For this review, take the finished solid that the model builds, in its own axes (mm). Coordinates: 2 decimals unless noted, no trailing zeros. Order: outer loops, then holes, each group sorted by start corner. A loop starts at its lowest first (then second) coordinate and runs counter-clockwise, first axis right, second up. Notation, with made-up numbers: M -17,-21 L 41,-21 A13 cw 41,-10 Z; hole C 68.25,-34 d5. An arc over 180 degrees is marked long. Use one line per item in the form item = value. Start each with the question number.
```python
from build123d import *

# Parameters (mm, degrees)
ESBO_O1_R                = 16
RESSALTO_EXTRUS_O1_DEPTH = 6
ESBO_O2_R                = 3
ESBO_O2_W                = 55
ESBO_O2_H                = 34
ESBO_O2_W_2              = 48
ESBO_O2_H_2              = 20
ESBO_O2_W_3              = 12.5
CORTE_EXTRUS_O1_DEPTH    = 215.755675129
RESSALTO_EXTRUS_O2_DEPTH = 6
ESBO_O4_R                = 3.5
CORTE_EXTRUS_O2_DEPTH    = 215.755675129
FILETE1_R                = 2
CHANFRO1_SIZE            = 8
CHANFRO2_SIZE            = 2
ESBO_O5_R                = 3.5
CORTE_EXTRUS_O3_DEPTH    = 215.755675129
CHANFRO3_SIZE            = 1
ESBO_O8_R                = 3
CORTE_EXTRUS_O5_DEPTH    = 215.755675129


with BuildPart() as part:
    # Esboço1 → Ressalto-extrusão1 (new body)
    with BuildSketch(Plane.XY):
        Polygon((0, 0), (0, 137), (41, 178), (79, 178), (120, 137), (120, 0), align=None)
        with Locations((60, 146.25)):
            Circle(ESBO_O1_R, mode=Mode.SUBTRACT)
    extrude(amount=RESSALTO_EXTRUS_O1_DEPTH)

    # Esboço2 → Corte-extrusão1 (cut, through all)
    with BuildSketch(Plane(origin=(0, 0, 0), x_dir=(-1, 0, 0), z_dir=(0, 0, -1))):
        with Locations((-60, 171.75)):
            Circle(ESBO_O2_R)
        with Locations((-34.5, 146.25)):
            Circle(ESBO_O2_R)
        with Locations((-60, 120.75)):
            Circle(ESBO_O2_R)
        with Locations((-85.5, 146.25)):
            Circle(ESBO_O2_R)
        with Locations((-60, 42.4)):
            Rectangle(ESBO_O2_W, ESBO_O2_H)
        Polygon((-56, 83.4), (-28, 83.4), (-28, 111.4), (-12, 111.4), (-12, 67.4), (-56, 67.4), align=None)
        with Locations((-60, 101.4)):
            Rectangle(ESBO_O2_W_2, ESBO_O2_H_2)
        with Locations((-18.25, 42.4)):
            Rectangle(ESBO_O2_W_3, ESBO_O2_H)
        Polygon((-64, 83.4), (-64, 67.4), (-108, 67.4), (-108, 111.4), (-92, 111.4), (-92, 83.4), align=None)
        with Locations((-101.75, 42.4)):
            Rectangle(ESBO_O2_W_3, ESBO_O2_H)
        with BuildLine():
            Line((-93.472953207, 152.213338294), (-108, 137.686291501))
            Line((-108, 137.686291501), (-108, 119.4))
            Line((-108, 119.4), (-80.858511452, 119.4))
            ThreePointArc((-80.858511452, 119.4), (-91.735718134, 134.049828095), (-93.472953207, 152.213338294))
        make_face()
        with BuildLine():
            Line((-26.527046793, 152.213338294), (-12, 137.686291501))
            Line((-12, 137.686291501), (-12, 119.4))
            Line((-12, 119.4), (-39.141488548, 119.4))
            ThreePointArc((-39.141488548, 119.4), (-28.264281866, 134.049828095), (-26.527046793, 152.213338294))
        make_face()
    extrude(amount=-CORTE_EXTRUS_O1_DEPTH, mode=Mode.SUBTRACT)

    # Esboço3 → Ressalto-extrusão2 (add, through all)
    with BuildSketch(Plane.XY.offset(6)):
        Polygon((28, 89.056854249), (12, 73.056854249), (12, 67.4), (17.656854249, 67.4), (33.656854249, 83.4), (28, 83.4), align=None)
        Polygon((86.343145751, 83.4), (102.343145751, 67.4), (108, 67.4), (108, 73.056854249), (92, 89.056854249), (92, 83.4), align=None)
    extrude(amount=-RESSALTO_EXTRUS_O2_DEPTH)

    # Esboço4 → Corte-extrusão2 (cut, through all)
    with BuildSketch(Plane.XY.offset(6)):
        with Locations((8, 12.7)):
            Circle(ESBO_O4_R)
        with Locations((33.4, 12.7)):
            Circle(ESBO_O4_R)
        with Locations((86.6, 12.7)):
            Circle(ESBO_O4_R)
        with Locations((112, 12.7)):
            Circle(ESBO_O4_R)
    extrude(amount=-CORTE_EXTRUS_O2_DEPTH, mode=Mode.SUBTRACT)

    # Filete1
    filete1_edges = [part.edges().sort_by_distance(p)[0] for p in [
        (39.141488548, 119.4, 3),
        (26.527046793, 152.213338294, 3),
        (12, 137.686291501, 3),
        (12, 119.4, 3),
        (108, 73.056854249, 3),
        (102.343145751, 67.4, 3),
        (17.656854249, 67.4, 3),
        (12, 73.056854249, 3),
        (93.472953207, 152.213338294, 3),
        (80.858511452, 119.4, 3),
        (108, 119.4, 3),
        (108, 137.686291501, 3),
    ]]
    fillet(filete1_edges, radius=FILETE1_R)

    # Chanfro1
    chanfro1_edges = [part.edges().sort_by_distance(p)[0] for p in [
        (87.5, 25.4, 3),
        (87.5, 59.4, 3),
        (32.5, 59.4, 3),
        (32.5, 25.4, 3),
    ]]
    chamfer(chanfro1_edges, length=CHANFRO1_SIZE)

    # Chanfro2
    chanfro2_edges = [part.edges().sort_by_distance(p)[0] for p in [
        (64, 83.4, 3),
        (64, 67.4, 3),
        (108, 111.4, 3),
        (92, 111.4, 3),
        (84, 91.4, 3),
        (84, 111.4, 3),
        (36, 111.4, 3),
        (36, 91.4, 3),
        (95.5, 25.4, 3),
        (108, 25.4, 3),
        (108, 59.4, 3),
        (95.5, 59.4, 3),
        (24.5, 25.4, 3),
        (24.5, 59.4, 3),
        (12, 59.4, 3),
        (12, 25.4, 3),
        (28, 111.4, 3),
        (12, 111.4, 3),
        (56, 67.4, 3),
        (56, 83.4, 3),
    ]]
    chamfer(chanfro2_edges, length=CHANFRO2_SIZE)

    # Esboço5 → Corte-extrusão3 (cut, through all)
    with BuildSketch(Plane.XY.offset(6)):
        with Locations((6.35, 128.4)):
            Circle(ESBO_O5_R)
        with Locations(Location((113.65, 128.4, 0), (0, 0, 180))):
            Circle(ESBO_O5_R)
    extrude(amount=-CORTE_EXTRUS_O3_DEPTH, mode=Mode.SUBTRACT)

    # Chanfro3
    chanfro3_edges = [part.edges().sort_by_distance(p)[0] for p in [
        (0, 0, 3),
        (120, 0, 3),
    ]]
    chamfer(chanfro3_edges, length=CHANFRO3_SIZE)

    # Esboço8 → Corte-extrusão5 (cut, through all)
    with BuildSketch(Plane.XY.offset(6)):
        with Locations((114, 34)):
            Circle(ESBO_O8_R)
    extrude(amount=-CORTE_EXTRUS_O5_DEPTH, mode=Mode.SUBTRACT)


solid = part.part
```
1. To check wall thickness, follow line 1 (Y direction, x = 60, z = 2.05); line 2 (Y direction, x = 86.6, z = 1.2); line 3 (X direction, y = 109.5, z = 1.25). State the ranges of each line that lie inside material, in increasing order.
2. Consider section B-B, the plane x = 49. Write out the cut boundary in (y, z), plus the area to 3 significant figures.
3. Consider section C-C, the plane y = 12.7. Write out the cut boundary in (x, z), plus the area to 3 significant figures.
4. Consider section D-D, the plane x = 6.35. Write out the cut boundary in (y, z), plus the area to 3 significant figures.
5. The part is to be moulded in two halves that separate along X. For faces 1 (the flat face through (108, 42, 3)), 2 (the flat face through (12, 42, 3)), 3 (the flat face through (0, 68, 3)), 4 (the flat face through (60, 178, 3)), say which applies: pulls with the +X half, pulls with the -X half, needs draft (parallel to the pull), parting line crosses it, or undercut.
6. For pin 1 Ø3 at (y, z) = (155.5, 3.5) entering from +X, flat-tipped, find the tip position at first contact; note if it passes through.
7. Consider section A-A, the plane y = 171.75. Write out the cut boundary in (x, z), plus the area to 3 significant figures.
Answers follow:
q1.line_1 = 0 to 25.4, 59.4 to 91.4, 111.4 to 117.75, 123.75 to 130.25, 162.25 to 168.75, 174.75 to 178
q1.line_2 = 0 to 9.2, 16.2 to 32.5, 52.3 to 67.4, 83.14 to 119.4, 125.07 to 143.46, 149.04 to 170.4
q1.line_3 = 0 to 12.1, 27.9 to 36.1, 83.9 to 92.1, 107.9 to 120
q2.outline = M 0,0 L 25.4,0 L 25.4,6 L 0,6 Z; M 59.4,0 L 67.4,0 L 67.4,6 L 59.4,6 Z; M 83.4,0 L 91.4,0 L 91.4,6 L 83.4,6 Z; M 111.4,0 L 134.63,0 L 134.63,6 L 111.4,6 Z; M 157.87,0 L 178,0 L 178,6 L 157.87,6 Z
q2.area = 509 mm²
q3.outline = M 0,0 L 4.5,0 L 4.5,6 L 0,6 Z; M 11.5,0 L 29.9,0 L 29.9,6 L 11.5,6 Z; M 36.9,0 L 83.1,0 L 83.1,6 L 36.9,6 Z; M 90.1,0 L 108.5,0 L 108.5,6 L 90.1,6 Z; M 115.5,0 L 120,0 L 120,6 L 115.5,6 Z
q3.area = 552 mm²
q4.outline = M 0,0 L 9.61,0 L 9.61,6 L 0,6 Z; M 15.79,0 L 124.9,0 L 124.9,6 L 15.79,6 Z; M 131.9,0 L 143.35,0 L 143.35,6 L 131.9,6 Z
q4.area = 781 mm²
q5.face_1 = undercut
q5.face_2 = undercut
q5.face_3 = pulls with the -X half
q5.face_4 = needs draft
q6.pin_1 = 103
q7.outline = M 34.75,0 L 57,0 L 57,6 L 34.75,6 Z; M 63,0 L 85.25,0 L 85.25,6 L 63,6 Z
q7.area = 267 mm²
